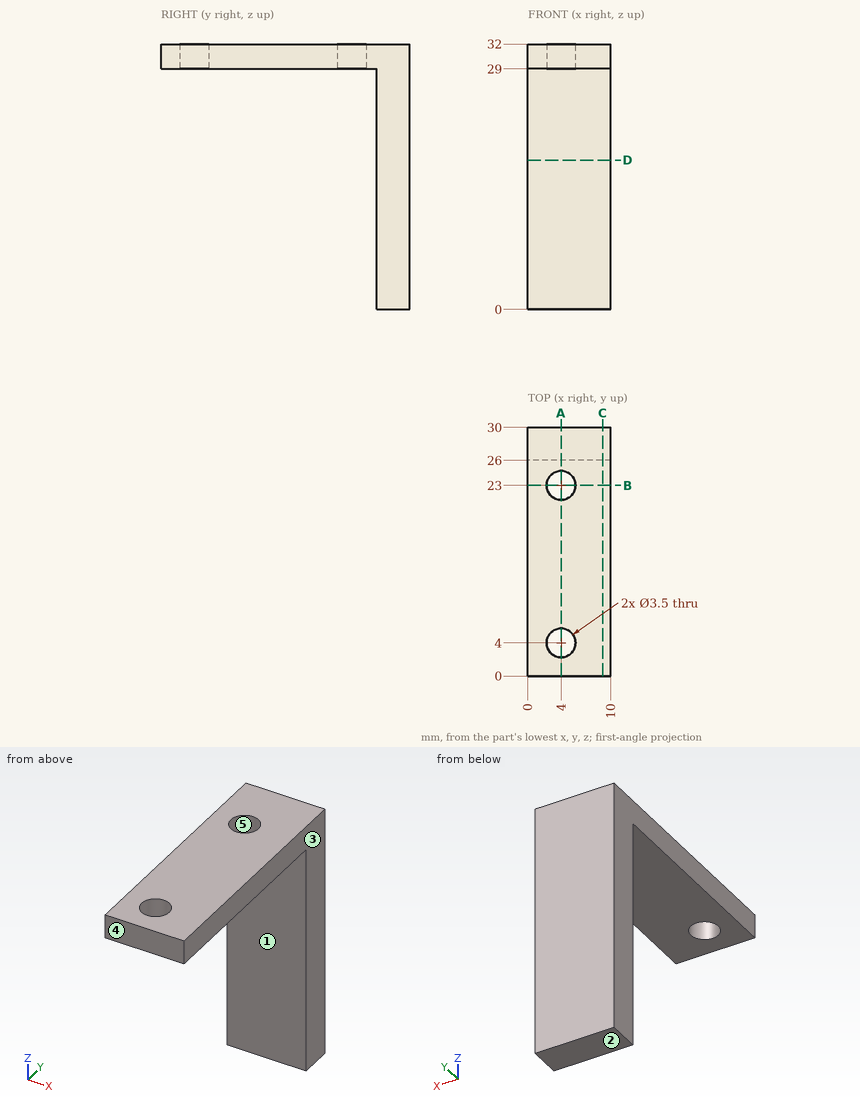
The drawing under review shows one solid part. Ordinate dimensions are in mm from its lowest x, y, z. A direction names the side the tool comes from. Round coordinates to 2 decimals unless told otherwise and drop trailing zeros. Write each loop counter-clockwise with the first axis right and the second up, starting at its lowest first coordinate (ties: lowest second). Pieces come first, ordered by that corner, then holes. Notation, with made-up numbers: (-24.75, -37) -> (26.25, -37) arc R21 cw to (26.25, -3) -> close; hole circle Ø8 at (79, 20.5). An arc over 180 degrees is marked (long way). One line per question, with ' | ' between items.
(1) Machinability: for the marked faces 1 and 2, which of the approach directions +Z, -Z, +X, -X, +Y, -Y give a long, thin tool a straight path to every point of the face, cutting with its end or side? Answer none if there is none.
Result sheet:
face 1: -Z, +X, -X, -Y | face 2: -Z, +X, -X, +Y, -Y
(2) Take a section at B-B, the plane y = 23. State the section outline as (x, z) points, and give its area (3 significant figures).
Result sheet:
outline: (0, 29) -> (2.25, 29) -> (2.25, 32) -> (0, 32) -> close; (5.75, 29) -> (10, 29) -> (10, 32) -> (5.75, 32) -> close | area: 19.5 mm2
(3) Take a section at C-C, the plane x = 9. State the section outline as (y, z) points, and give its area (3 significant figures).
Result sheet:
outline: (0, 29) -> (26, 29) -> (26, 0) -> (30, 0) -> (30, 32) -> (0, 32) -> close | area: 206 mm2
(4) Wall thickness on line 1 (Y direction, x = 4, z = 31.3); line 2 (X direction, y = 23, z = 29.75); line 3 (Y direction, x = 7, z = 13.5): over which ranges is each line inside the solid? List them lowest first. Write a range as [from, to].
Result sheet:
line 1: [0, 2.25], [5.75, 21.25], [24.75, 30] | line 2: [0, 2.25], [5.75, 10] | line 3: [26, 30]
(5) Take a section at A-A, the plane x = 4. State the section outline as (y, z) points.
Result sheet:
outline: (0, 29) -> (2.25, 29) -> (2.25, 32) -> (0, 32) -> close; (5.75, 29) -> (21.25, 29) -> (21.25, 32) -> (5.75, 32) -> close; (24.75, 29) -> (26, 29) -> (26, 0) -> (30, 0) -> (30, 32) -> (24.75, 32) -> close
(6) Take a section at D-D, the plane z = 18. State the section outline as (x, y) points.
Result sheet:
outline: (0, 26) -> (10, 26) -> (10, 30) -> (0, 30) -> close
(7) Draft analysis for pull direction Y (two halves, no side actions). For the marked faces 3, 4 and 5, state which applies: released by +Y, released by -Y, zero draft, split by the parting line, or undercut.
Result sheet:
face 3: zero draft | face 4: released by -Y | face 5: undercut
(8) Insertion check: P1, Ø3, axis at x = 4, z = 4.5, coming from the -Y side; P2, Ø5.5, axis at x = 4, y = 23, coming from the -Z side; P3, Ø3, axis at y = 24, z = 16.5, coming from the -X side. Each pin has a flat end and moves straight along its axis. Give the tip position at first contact, or say it passes through.
Result sheet:
P1: y = 26 | P2: z = 29 | P3: through
